Geometry check sheet. Reference: the model listing, model coordinates, mm. Face numbers are marked on the shaded views. Coordinates: 2 decimals unless noted, no trailing zeros. Loops run counter-clockwise (first coordinate to the right, second up) from the corner with the lowest first, then second, coordinate; pieces in that order, holes last.
from build123d import *

# Parameters (mm, degrees)
SPLIT_SADDLE_WITH_37_0_MM_PROTOTYPE_BORE_DEPTH = 14
M4_THROUGH_HOLES_DEPTH                         = 44.144988121
M4_THROUGH_HOLES_DEPTH_BACK                    = 44.144988121
SKETCH2_R                                      = 2.25


with BuildPart() as part:
    # Split saddle with 37.0 mm prototype  2 → Split saddle with 37.0 mm prototype bore (new body)
    with BuildSketch(Plane.XY):
        with BuildLine():
            Line((-29.5, 7), (29.5, 7))
            Line((29.5, 7), (29.5, 28.2))
            Line((29.5, 28.2), (18.497567408, 28.2))
            ThreePointArc((18.497567408, 28.2), (0, 10), (-18.497567408, 28.2))
            Line((-18.497567408, 28.2), (-29.5, 28.2))
            Line((-29.5, 28.2), (-29.5, 7))
        make_face()
    extrude(amount=SPLIT_SADDLE_WITH_37_0_MM_PROTOTYPE_BORE_DEPTH)

    # Sketch2 → M4 through holes (cut, two sides: drawn at the far end of the back side and taken through both)
    with BuildSketch(Plane(origin=(0, 0, 0), x_dir=(1, 0, 0), z_dir=(0, 1, 0)).offset(-M4_THROUGH_HOLES_DEPTH_BACK)):
        with Locations(Location((-24.5, -7, 0), (0, 0, 270))):
            Circle(SKETCH2_R)
        with Locations(Location((24.5, -7, 0), (0, 0, 270))):
            Circle(SKETCH2_R)
    extrude(amount=M4_THROUGH_HOLES_DEPTH + M4_THROUGH_HOLES_DEPTH_BACK, mode=Mode.SUBTRACT)


solid = part.part
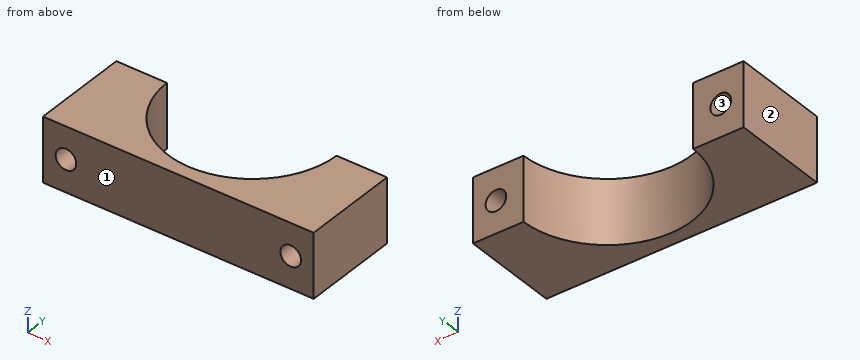
(1) Draft check along X on the marked faces 1, 2 and 3. Enter one of: +X half, -X half, draft (parallel to the pull), parting line (faces both ways), or undercut.
Findings:
face 1: draft
face 2: -X half
face 3: undercut
(2) Gauge pin test, flat ends, axial feed: pin 1 Ø2 at (x, z) = (-4.5, 10.5) entering from +Y; pin 2 Ø2.5 at (x, z) = (-24.5, 7) entering from -Y. Record the tip position at first contact, or that the pin passes through.
Findings:
pin 1: stops at y = 10.84
pin 2: passes through
(3) Sectioned sample at D-D on y = 20.5. Record the cut outline in (x, z).
Findings:
outline: (-29.5, 0) - (-16.68, 0) - (-16.68, 14) - (-29.5, 14) - close; (16.68, 0) - (29.5, 0) - (29.5, 14) - (16.68, 14) - close; hole circle Ø4.5 at (-24.5, 7); hole circle Ø4.5 at (24.5, 7)
(4) Scan lines: L1, parallel to X at y = 17, z = 7; L2, parallel to X at y = 13.5, z = 7; L3, parallel to Z at x = -24.5, y = 21.75. Record each from-to range of solid material in increasing order.
Findings:
L1: x = -29.5 to -26.75, -22.25 to -14.49, 14.49 to 22.25, 26.75 to 29.5
L2: x = -29.5 to -26.75, -22.25 to -10.83, 10.83 to 22.25, 26.75 to 29.5
L3: z = 0 to 4.75, 9.25 to 14
(5) Sectioned sample at A-A on y = 13.5. Record the cut outline in (x, z), and give its area (3 significant figures).
Findings:
outline: (-29.5, 0) - (-10.83, 0) - (-10.83, 14) - (-29.5, 14) - close; (10.83, 0) - (29.5, 0) - (29.5, 14) - (10.83, 14) - close; hole circle Ø4.5 at (-24.5, 7); hole circle Ø4.5 at (24.5, 7)
area: 491 mm2
(6) Sectioned sample at B-B on x = 24.5. Record the cut outline in (y, z).
Findings:
outline: (7, 0) - (28.2, 0) - (28.2, 4.75) - (7, 4.75) - close; (7, 9.25) - (28.2, 9.25) - (28.2, 14) - (7, 14) - close
